from build123d import *

# Parameters (mm, degrees)
F0_R     = 3.90525
F1_DEPTH = 7.62
F2_W     = 9.525
F2_H     = 9.525
F3_DEPTH = 3.175
F6_R     = 0.508
F7_SIZE  = 1.778


with BuildPart() as f1:
    # F0 (on Top) → F1 (new body)
    with BuildSketch(Plane.XY):
        Circle(F0_R)
    extrude(amount=-F1_DEPTH)

    # F2 (on face) → F3 (join)
    with BuildSketch(Plane.XY):
        Rectangle(F2_W, F2_H)
    extrude(amount=F3_DEPTH)

    # F4 (on Front) → F5 (revolve, cut)
    with BuildSketch(Plane.XZ):
        Polygon((0, 1.5875), (4.572, 3.175), (0, 3.175), align=None)
    revolve(axis=Axis((0, 0, 2.38125), (0, 0, 1)), mode=Mode.SUBTRACT)

    # F6
    f6_edges = [f1.edges().sort_by_distance(p)[0] for p in [
        (-4.7625, 4.7625, 1.5875),
        (4.7625, 4.7625, 1.5875),
        (-4.7625, -4.7625, 1.5875),
        (4.7625, -4.7625, 1.5875),
    ]]
    fillet(f6_edges, radius=F6_R)

    # F7
    f7_edges = [f1.edges().sort_by_distance(p)[0] for p in [
        (-3.90525, 0, -7.62),
    ]]
    chamfer(f7_edges, length=F7_SIZE)


solid = f1.part
Geometry check sheet. Reference: the model listing, model coordinates, mm. A direction names the side the tool comes from. Round coordinates to 2 decimals unless told otherwise and drop trailing zeros. Write each loop counter-clockwise with the first axis right and the second up, starting at its lowest first coordinate (ties: lowest second). Pieces come first, ordered by that corner, then holes.
Item 1: Access from +Z, -Z, +X, -X, +Y, -Y to the whole of each face (thin tool, end or side, straight path). Record for faces 1 (the face through (-4.3, 0.1, 0)), 2 (the face through (0, 0, -7.62)).
Determined:
face 1: -Z
face 2: -Z, +X, -X, +Y, -Y
Item 2: Material ranges on line 1 along Z through (x, y) = (4, -3.75) (3 decimals); line 2 along X through (y, z) = (2.25, -2); line 3 along Z through (x, y) = (0.75, 0.75), recorded low to high.
Determined:
line 1: z = 0 to 3.175
line 2: x = -3.19 to 3.19
line 3: z = -7.62 to 1.96
Item 3: Mould release check, pull along X, two halves, no side actions. Record for faces 3 (the face through (-0.51, 3.87, -2.88)), 4 (the face through (0.273, 0.086, 1.687)), 5 (the face through (-1.1, -4.6, 3.175)): +X half, -X half, draft (parallel to the pull), parting line (faces both ways), or undercut.
Determined:
face 3: parting line
face 4: undercut
face 5: draft
Item 4: Section check A-A (z = -2). Record the boundary of the cut face in (x, y).
Determined:
outline: circle Ø7.81 at (0, 0)
Item 5: Section check B-B (z = -6.25). Record the boundary of the cut face in (x, y), plus the area to 3 significant figures.
Determined:
outline: circle Ø6.99 at (0, 0)
area: 38.4 mm2
Item 6: Go/stop test with flat-tipped pins: pin 1 Ø1 at (x, z) = (3, -2.5) entering from -Y; pin 2 Ø2 at (x, z) = (-2.5, -5) entering from -Y; pin 3 Ø1 at (x, y) = (-1, 1.5) entering from +Z. Record where each tip stops, or that it passes through.
Determined:
pin 1: stops at y = -3
pin 2: stops at y = -3.61
pin 3: stops at z = 2.39
